CAD build for the part. Positions are in the model's coordinates, mm. Face numbers are marked on the shaded views. A direction names the side the tool comes from. Give positions to 0.01 mm unless a question says otherwise; leave off trailing zeros. Loops run counter-clockwise (first coordinate to the right, second up) from the corner with the lowest first, then second, coordinate; pieces in that order, holes last.
Item 1: Saw through at B-B on y = 0. Give the cut face in (x, z).
Item 2: Saw through at A-A on z = -8. Give the cut face in (x, y), plus the area to 3 significant figures.
Item 3: Saw through at C-C on x = 8. Give the cut face in (y, z).
Item 4: Drop flat-ended pins along their axis: P1, Ø5.5, axis at x = 0, z = -32, coming from the +Y side; P2, Ø3, axis at x = 0.5, z = -1, coming from the -Y side; P3, Ø3, axis at x = 0, z = -16, coming from the -Y side; P4, Ø2, axis at y = -1.5, z = -20.5, coming from the +X side. Give the stop position or say it passes through.
Item 5: Which spindle directions (+Z, -Z, +X, -X, +Y, -Y) get a long thin tool onto all of the face, cutting with end or side? Do the marked faces 1 and 2. Say none if no direction does.
Item 6: Probe probe 1 along X at (y, z) = (3.45, 0); probe 2 along X at (y, z) = (-2.5, -0.5); probe 3 along X at (y, z) = (-0.5, -24). List the from-to ranges inside material, lowest first.
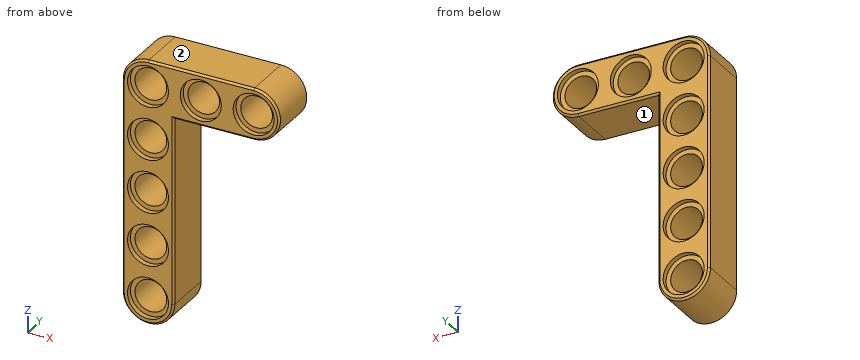
from build123d import *

# Parameters (mm, degrees)
BOSS_EXTRUDE1_DEPTH       = 3.9
FILLET1_R                 = 3.9
SKETCH2_R                 = 2.4
CUT_EXTRUDE2_DEPTH        = 42.781096204
SKETCH4_R                 = 3.1
CUT_EXTRUDE3_DEPTH        = 0.8
LPATTERN1_COUNT           = 5
LPATTERN1_PITCH           = 8
LPATTERN1_COPY_1_SKETCH_R = 3.1
LPATTERN1_COPY_1_DEPTH    = 0.8
LPATTERN1_COPY_2_SKETCH_R = 3.1
LPATTERN1_COPY_2_DEPTH    = 0.8
LPATTERN1_COPY_3_SKETCH_R = 3.1
LPATTERN1_COPY_3_DEPTH    = 0.8
LPATTERN1_COPY_4_SKETCH_R = 3.1
LPATTERN1_COPY_4_DEPTH    = 0.8
LPATTERN2_COUNT           = 3
LPATTERN2_PITCH           = 8
LPATTERN2_COPY_1_SKETCH_R = 3.1
LPATTERN2_COPY_1_DEPTH    = 0.8
LPATTERN2_COPY_2_SKETCH_R = 3.1
LPATTERN2_COPY_2_DEPTH    = 0.8
CHAMFER1_SIZE             = 0.3


with BuildPart() as part:
    # Sketch1 → Boss-Extrude1 (new, symmetric)
    with BuildSketch(Plane(origin=(0, 0, 0), x_dir=(1, 0, 0), z_dir=(0, 1, 0))):
        with BuildLine():
            Line((3.9, 3.9), (16, 3.9))
            ThreePointArc((16, 3.9), (19.9, 0), (16, -3.9))
            Line((16, -3.9), (-3.9, -3.9))
            Line((-3.9, -3.9), (-3.9, 32))
            ThreePointArc((-3.9, 32), (0, 35.9), (3.9, 32))
            Line((3.9, 32), (3.9, 3.9))
        make_face()
    extrude(amount=BOSS_EXTRUDE1_DEPTH, both=True)

    # Fillet1
    fillet1_edges = [part.edges().sort_by_distance(p)[0] for p in [
        (-3.9, 0, 3.9),
    ]]
    fillet(fillet1_edges, radius=FILLET1_R)

    # Sketch2 → Cut-Extrude2 (cut, through all)
    with BuildSketch(Plane(origin=(0, 3.9, 0), x_dir=(1, 0, 0), z_dir=(0, 1, 0))):
        with Locations(Location((0, 0, 0), (0, 0, 270))):
            Circle(SKETCH2_R)
    cut_extrude2 = extrude(amount=-CUT_EXTRUDE2_DEPTH, mode=Mode.SUBTRACT)

    # Sketch4 → Cut-Extrude3 (cut)
    with BuildSketch(Plane(origin=(0, 3.9, 0), x_dir=(1, 0, 0), z_dir=(0, 1, 0))):
        with Locations(Location((0, 0, 0), (0, 0, 270))):
            Circle(SKETCH4_R)
    cut_extrude3 = extrude(amount=-CUT_EXTRUDE3_DEPTH, mode=Mode.SUBTRACT)

    # Mirror1: Cut-Extrude3 across plane
    add(cut_extrude3.mirror(Plane.ZX), mode=Mode.SUBTRACT)

    # LPattern1: Cut-Extrude2, Cut-Extrude3 ×5
    with Locations(*[(0, 0, -i * LPATTERN1_PITCH) for i in range(1, LPATTERN1_COUNT)]):
        add(cut_extrude2, mode=Mode.SUBTRACT)
        add(cut_extrude3, mode=Mode.SUBTRACT)

    # LPattern1 copy 1 sketch → LPattern1 copy 1 (cut)
    with BuildSketch(Plane(origin=(0, -3.9, -8), x_dir=(1, 0, 0), z_dir=(0, -1, 0))):
        Circle(LPATTERN1_COPY_1_SKETCH_R)
    extrude(amount=-LPATTERN1_COPY_1_DEPTH, mode=Mode.SUBTRACT)

    # LPattern1 copy 2 sketch → LPattern1 copy 2 (cut)
    with BuildSketch(Plane(origin=(0, -3.9, -16), x_dir=(1, 0, 0), z_dir=(0, -1, 0))):
        Circle(LPATTERN1_COPY_2_SKETCH_R)
    extrude(amount=-LPATTERN1_COPY_2_DEPTH, mode=Mode.SUBTRACT)

    # LPattern1 copy 3 sketch → LPattern1 copy 3 (cut)
    with BuildSketch(Plane(origin=(0, -3.9, -24), x_dir=(1, 0, 0), z_dir=(0, -1, 0))):
        Circle(LPATTERN1_COPY_3_SKETCH_R)
    extrude(amount=-LPATTERN1_COPY_3_DEPTH, mode=Mode.SUBTRACT)

    # LPattern1 copy 4 sketch → LPattern1 copy 4 (cut)
    with BuildSketch(Plane(origin=(0, -3.9, -32), x_dir=(1, 0, 0), z_dir=(0, -1, 0))):
        Circle(LPATTERN1_COPY_4_SKETCH_R)
    extrude(amount=-LPATTERN1_COPY_4_DEPTH, mode=Mode.SUBTRACT)

    # LPattern2: Cut-Extrude2, Cut-Extrude3 ×3
    with Locations(*[(i * LPATTERN2_PITCH, 0, 0) for i in range(1, LPATTERN2_COUNT)]):
        add(cut_extrude2, mode=Mode.SUBTRACT)
        add(cut_extrude3, mode=Mode.SUBTRACT)

    # LPattern2 copy 1 sketch → LPattern2 copy 1 (cut)
    with BuildSketch(Plane(origin=(8, -3.9, 0), x_dir=(1, 0, 0), z_dir=(0, -1, 0))):
        Circle(LPATTERN2_COPY_1_SKETCH_R)
    extrude(amount=-LPATTERN2_COPY_1_DEPTH, mode=Mode.SUBTRACT)

    # LPattern2 copy 2 sketch → LPattern2 copy 2 (cut)
    with BuildSketch(Plane(origin=(16, -3.9, 0), x_dir=(1, 0, 0), z_dir=(0, -1, 0))):
        Circle(LPATTERN2_COPY_2_SKETCH_R)
    extrude(amount=-LPATTERN2_COPY_2_DEPTH, mode=Mode.SUBTRACT)

    # Chamfer1
    chamfer1_edges = [part.edges().sort_by_distance(p)[0] for p in [
        (-3.9, 3.9, -16),
        (8, -3.9, 3.9),
        (8, 3.9, 3.9),
        (19.9, 3.9, 0),
        (-2.757716447, -3.9, 2.757716447),
        (-2.757716447, 3.9, 2.757716447),
        (9.95, 3.9, -3.9),
        (3.9, 3.9, -17.95),
        (9.95, -3.9, -3.9),
        (19.9, -3.9, 0),
        (-3.9, -3.9, -16),
        (0, -3.9, -35.9),
        (3.9, -3.9, -17.95),
        (0, 3.9, -35.9),
    ]]
    chamfer(chamfer1_edges, length=CHAMFER1_SIZE)


solid = part.part
Results below:
1. outline: (-3.9, -32) arc R3.9 ccw to (3.9, -32) - (3.9, -3.9) - (16, -3.9) arc R3.9 ccw to (16, 3.9) - (0, 3.9) arc R3.9 ccw to (-3.9, 0) - close; hole circle Ø4.8 at (0, -32); hole circle Ø4.8 at (0, -24); hole circle Ø4.8 at (0, -16); hole circle Ø4.8 at (0, -8); hole circle Ø4.8 at (0, 0); hole circle Ø4.8 at (8, 0); hole circle Ø4.8 at (16, 0)
2. outline: (-3.9, -3.6) - (-3.6, -3.9) - (-3.1, -3.9) - (-3.1, -3.1) - (-2.4, -3.1) - (-2.4, 3.1) - (-3.1, 3.1) - (-3.1, 3.9) - (-3.6, 3.9) - (-3.9, 3.6) - close; (2.4, -3.1) - (3.1, -3.1) - (3.1, -3.9) - (3.6, -3.9) - (3.9, -3.6) - (3.9, 3.6) - (3.6, 3.9) - (3.1, 3.9) - (3.1, 3.1) - (2.4, 3.1) - close
2. area: 21.0 mm2
3. outline: (-3.9, -3.6) - (-3.6, -3.9) - (3.6, -3.9) - (3.9, -3.6) - (3.9, -3.1) - (3.1, -3.1) - (3.1, -2.4) - (-3.1, -2.4) - (-3.1, -3.1) - (-3.9, -3.1) - close; (-3.9, 3.1) - (-3.1, 3.1) - (-3.1, 2.4) - (3.1, 2.4) - (3.1, 3.1) - (3.9, 3.1) - (3.9, 3.6) - (3.6, 3.9) - (-3.6, 3.9) - (-3.9, 3.6) - close
4. P1: stops at y = 3.1
4. P2: stops at y = -3.1
4. P3: passes through
4. P4: stops at x = 3.9
5. face 1: -Z, +X, +Y, -Y
5. face 2: +Z, +X, -X, +Y, -Y
6. probe 1: x = -3.9 to -3.1, 3.1 to 4.9, 11.1 to 12.9, 19.1 to 19.9
6. probe 2: x = -3.9 to -2.35, 2.35 to 5.65, 10.35 to 13.65, 18.35 to 19.87
6. probe 3: x = -3.9 to -2.4, 2.4 to 3.9
